from build123d import *

# Parameters (mm, degrees)
ESBO_O1_W                = 45
ESBO_O1_H                = 45
ESBO_O1_R                = 1.75
ESBO_O1_R_2              = 11.5
RESSALTO_EXTRUS_O1_DEPTH = 5
ESBO_O3_R                = 4
RESSALTO_EXTRUS_O2_DEPTH = 45
RESSALTO_EXTRUS_O3_DEPTH = 10
ESBO_O5_R                = 1.75
CORTE_EXTRUS_O2_DEPTH    = 15


with BuildPart() as part:
    # Esboço1 → Ressalto-extrusão1 (new body)
    with BuildSketch(Plane.XY):
        Rectangle(ESBO_O1_W, ESBO_O1_H)
        with Locations((-15.5, 15.5)):
            Circle(ESBO_O1_R, mode=Mode.SUBTRACT)
        with Locations((15.5, 15.5)):
            Circle(ESBO_O1_R, mode=Mode.SUBTRACT)
        with Locations((15.5, -15.5)):
            Circle(ESBO_O1_R, mode=Mode.SUBTRACT)
        with Locations((-15.5, -15.5)):
            Circle(ESBO_O1_R, mode=Mode.SUBTRACT)
        Circle(ESBO_O1_R_2, mode=Mode.SUBTRACT)
    extrude(amount=RESSALTO_EXTRUS_O1_DEPTH)

    # Esboço3 → Ressalto-extrusão2 (add)
    # profile 1 of 2: a face of its own
    with BuildSketch(Plane.ZY.offset(22.5)):
        with BuildLine():
            Line((0, 30), (0, 21.937742252))
            Line((0, 21.937742252), (5, 21.937742252))
            ThreePointArc((5, 21.937742252), (16.64852927, 34.74341649), (0, 30))
        make_face()
        with Locations(Location((9, 30, 0), (0, 0, 270))):
            Circle(ESBO_O3_R, mode=Mode.SUBTRACT)
    # profile 2 of 2: a face of its own
    with BuildSketch(Plane.ZY.offset(22.5)):
        with BuildLine():
            Line((5, -21.937742252), (0, -21.937742252))
            Line((0, -21.937742252), (0, -30))
            ThreePointArc((0, -30), (16.64852927, -34.74341649), (5, -21.937742252))
        make_face()
        with Locations(Location((9, -30, 0), (0, 0, 270))):
            Circle(ESBO_O3_R, mode=Mode.SUBTRACT)
    extrude(amount=-RESSALTO_EXTRUS_O2_DEPTH)

    # Esboço4 → Ressalto-extrusão3 (add)
    # profile 1 of 2: a face of its own
    with BuildSketch(Plane.ZY.offset(22.5)):
        Polygon((7.247929139, 38.827811037), (-7, 36), (-7, 24), (0, 22.610697943), align=None)
        Polygon((0, 30), (0, 32.8), (-3.5, 32.8), (-3.5, 27.2), (0, 27.2), align=None, mode=Mode.SUBTRACT)
    # profile 2 of 2: a face of its own
    with BuildSketch(Plane.ZY.offset(22.5)):
        Polygon((7.247929139, -38.827811037), (0, -22.610697943), (-7, -24), (-7, -36), align=None)
        Polygon((0, -27.2), (0, -30), (0, -32.8), (-3.5, -32.8), (-3.5, -27.2), align=None, mode=Mode.SUBTRACT)
    extrude(amount=-RESSALTO_EXTRUS_O3_DEPTH)

    # Esboço5 → Corte-extrusão2 (cut)
    with BuildSketch(Plane(origin=(0, 0, -7), x_dir=(-1, 0, 0), z_dir=(0, 0, -1))):
        with Locations((17.5, 30)):
            Circle(ESBO_O5_R)
        with Locations((17.5, -30)):
            Circle(ESBO_O5_R)
    extrude(amount=-CORTE_EXTRUS_O2_DEPTH, mode=Mode.SUBTRACT)


solid = part.part
CAD build for the part. Positions are in the model's coordinates, mm. A direction names the side the tool comes from. Round coordinates to 2 decimals unless told otherwise and drop trailing zeros. Loops run counter-clockwise (first coordinate to the right, second up) from the corner with the lowest first, then second, coordinate; pieces in that order, holes last.
(1) Wall check: line 1 along Z through (x, y) = (8, 30); line 2 along X through (y, z) = (30, 4.3); line 3 along Y through (x, z) = (-17.5, -6.25). Give the ranges that are in metal, low to high.
(2) Cut at A-A (x = 15.5). Give the cut face in (y, z).
(3) Drop flat-ended pins along their axis: pin 1 (3 mm diameter, centred on x = -19, z = -1, fed in from +Y); pin 2 (3 mm diameter, centred on x = 15.5, y = 15.5, fed in from +Z); pin 3 (4 mm diameter, centred on x = -16, z = -2, fed in from +Y); pin 4 (1.8 mm diameter, centred on x = -16.5, z = -2.5, fed in from -Y). Give the stop position or say it passes through.
(4) Cut at B-B (y = 15.5). Give the cut face in (x, z), plus the area to 3 significant figures.
(5) Which spindle directions (+Z, -Z, +X, -X, +Y, -Y) get a long thin tool onto all of the face, cutting with end or side? Do faces 5 (the cylindrical face through (-15.75, 30.08, 2.66)), 6 (the flat face through (-17.57, 23.315, -3.549)), 7 (the flat face through (-18, 28, -3.5)). Say none if no direction does.
(6) Two-plate mould, pull along Y, no slides. Class faces 1 (the cylindrical face through (-0.32, -35.02, 16.47)), 2 (the flat face through (-17.57, 37.434, 0.224)), 3 (the flat face through (-22.5, 1, 3)), 4 (the cylindrical face through (-16.11, -31.06, -5.27)): +Y half, -Y half, draft (parallel to the pull), parting line (faces both ways), or undercut.
(7) Cut at D-D (z = 15.5). Give the cut face in (x, y), plus the area to 3 significant figures.
(8) Cut at C-C (x = 10.5). Give the cut face in (y, z), plus the area to 3 significant figures.
Findings below:
1. line 1: z = 0 to 5, 13 to 18
1. line 2: x = -22.5 to -19.25, -15.75 to 22.5
1. line 3: y = -36.15 to -31.75, -28.25 to -23.85, 23.85 to 28.25, 31.75 to 36.15
2. outline: (-30, 0) - (-17.25, 0) - (-17.25, 5) - (-21.94, 5) arc R9 ccw (long way) to start; (-13.75, 0) - (13.75, 0) - (13.75, 5) - (-13.75, 5) - close; (17.25, 0) - (30, 0) arc R9 ccw (long way) to (21.94, 5) - (17.25, 5) - close; hole circle Ø8 at (-30, 9); hole circle Ø8 at (30, 9)
3. pin 1: stops at y = 37.49
3. pin 2: passes through
3. pin 3: stops at y = 37.39
3. pin 4: stops at y = -37.07
4. outline: (-22.5, 0) - (-17.25, 0) - (-17.25, 5) - (-22.5, 5) - close; (-13.75, 0) - (13.75, 0) - (13.75, 5) - (-13.75, 5) - close; (17.25, 0) - (22.5, 0) - (22.5, 5) - (17.25, 5) - close
4. area: 190 mm2
5. face 5: -Z
5. face 6: -Z, +X, -X
5. face 7: +X, -X
6. face 1: undercut
6. face 2: +Y half
6. face 3: draft
6. face 4: undercut
7. outline: (-22.5, -36.22) - (22.5, -36.22) - (22.5, -23.78) - (-22.5, -23.78) - close; (-22.5, 23.78) - (22.5, 23.78) - (22.5, 36.22) - (-22.5, 36.22) - close
7. area: 1,120 mm2
8. outline: (-30, 0) - (-4.69, 0) - (-4.69, 5) - (-21.94, 5) arc R9 ccw (long way) to start; (4.69, 0) - (30, 0) arc R9 ccw (long way) to (21.94, 5) - (4.69, 5) - close; hole circle Ø8 at (-30, 9); hole circle Ø8 at (30, 9)
8. area: 604 mm2
